from build123d import *

# Parameters (mm, degrees)
SKETCH1_R           = 2.38125
SKETCH1_R_2         = 14.2875
BOSS_EXTRUDE1_DEPTH = 6.35
FILLET1_R           = 12.7
SKETCH2_R           = 2.38125
CUT_EXTRUDE1_DEPTH  = 7.35
FILLET2_R           = 2.54


with BuildPart() as part:
    # Sketch1 → Boss-Extrude1 (new body)
    with BuildSketch(Plane(origin=(0, 0, 0), x_dir=(1, 0, 0), z_dir=(0, 1, 0))):
        Polygon((0, 0), (50.8, 0), (50.8, 127), (-25.4, 127), (-25.4, 50.8), (0, 50.8), align=None)
        with Locations((12.7, 12.7)):
            Circle(SKETCH1_R, mode=Mode.SUBTRACT)
        with Locations((25.4, 12.7)):
            Circle(SKETCH1_R, mode=Mode.SUBTRACT)
        with Locations((38.1, 12.7)):
            Circle(SKETCH1_R, mode=Mode.SUBTRACT)
        with Locations((25.4, 25.4)):
            Circle(SKETCH1_R, mode=Mode.SUBTRACT)
        with Locations((38.1, 25.4)):
            Circle(SKETCH1_R, mode=Mode.SUBTRACT)
        with Locations((25.4, 38.1)):
            Circle(SKETCH1_R, mode=Mode.SUBTRACT)
        with Locations((38.1, 38.1)):
            Circle(SKETCH1_R, mode=Mode.SUBTRACT)
        with Locations((12.7, 25.4)):
            Circle(SKETCH1_R, mode=Mode.SUBTRACT)
        with Locations((12.7, 38.1)):
            Circle(SKETCH1_R, mode=Mode.SUBTRACT)
        with Locations((6.35, 88.9)):
            Circle(SKETCH1_R_2, mode=Mode.SUBTRACT)
        with Locations((12.7, 50.8)):
            Circle(SKETCH1_R, mode=Mode.SUBTRACT)
        with Locations((25.4, 50.8)):
            Circle(SKETCH1_R, mode=Mode.SUBTRACT)
        with Locations((38.1, 50.8)):
            Circle(SKETCH1_R, mode=Mode.SUBTRACT)
    extrude(amount=BOSS_EXTRUDE1_DEPTH)

    # Fillet1
    fillet1_edges = [part.edges().sort_by_distance(p)[0] for p in [
        (-25.4, 3.175, -127),
        (50.8, 3.175, -127),
    ]]
    fillet(fillet1_edges, radius=FILLET1_R)

    # Sketch2 → Cut-Extrude1 (cut, through all)
    with BuildSketch(Plane(origin=(0, 6.35, 0), x_dir=(1, 0, 0), z_dir=(0, 1, 0))):
        with Locations((-19.05, 88.9)):
            Circle(SKETCH2_R)
        with Locations((-11.610512242, 106.860512242)):
            Circle(SKETCH2_R)
        with Locations((6.35, 114.3)):
            Circle(SKETCH2_R)
        with Locations((24.310512242, 106.860512242)):
            Circle(SKETCH2_R)
        with Locations((31.75, 88.9)):
            Circle(SKETCH2_R)
        with Locations((24.310512242, 70.939487758)):
            Circle(SKETCH2_R)
        with Locations((6.35, 63.5)):
            Circle(SKETCH2_R)
        with Locations((-11.610512242, 70.939487758)):
            Circle(SKETCH2_R)
    extrude(amount=-CUT_EXTRUDE1_DEPTH, mode=Mode.SUBTRACT)

    # Fillet2
    fillet2_edges = [part.edges().sort_by_distance(p)[0] for p in [
        (-25.4, 3.175, -50.8),
    ]]
    fillet(fillet2_edges, radius=FILLET2_R)


solid = part.part
Geometry check sheet. Reference: the model listing, model coordinates, mm. A direction names the side the tool comes from. Round coordinates to 2 decimals unless told otherwise and drop trailing zeros. Loops run counter-clockwise (first coordinate to the right, second up) from the corner with the lowest first, then second, coordinate; pieces in that order, holes last. Notation, with made-up numbers: (85.5, 38) - (93.5, 38) arc R28 cw to (93.5, 70) - close; hole circle Ø8 at (38, 59.25). An arc over 180 degrees is marked (long way). Answer as CSV lines item,"result".
(1) Depth check by flat-ended pin: pin 1 Ø4.5 at (x, z) = (12.7, -25.4) entering from +Y. Enter the tip coordinate at first touch or a pass-through.
Output values:
pin 1,"passes through"
(2) Cross-section at B-B, the plane z = -63.5. Enter the section's corners in (x, y), and give its area (3 significant figures).
Output values:
outline,"(-25.4, 0) - (3.97, 0) - (3.97, 6.35) - (-25.4, 6.35) - close; (8.73, 0) - (50.8, 0) - (50.8, 6.35) - (8.73, 6.35) - close"
area,"454 mm²"
(3) Cross-section at A-A, the plane x = 31.75. Enter the section's corners in (y, z).
Output values:
outline,"(0, -127) - (6.35, -127) - (6.35, -91.28) - (0, -91.28) - close; (0, -86.52) - (6.35, -86.52) - (6.35, 0) - (0, 0) - close"
(4) Cross-section at C-C, the plane z = -12.7. Enter the section's corners in (x, y).
Output values:
outline,"(0, 0) - (10.32, 0) - (10.32, 6.35) - (0, 6.35) - close; (15.08, 0) - (23.02, 0) - (23.02, 6.35) - (15.08, 6.35) - close; (27.78, 0) - (35.72, 0) - (35.72, 6.35) - (27.78, 6.35) - close; (40.48, 0) - (50.8, 0) - (50.8, 6.35) - (40.48, 6.35) - close"
(5) Release check for a two-part mould opening along X. For faces 1 (the face through (-24.636, 3.219, -51.524)), 2 (the face through (21, 6.35, -64)), 3 (the face through (12.39, 3.13, -53.16)) record: released by +X, released by -X, zero draft, split by the parting line, or undercut.
Output values:
face 1,"released by -X"
face 2,"zero draft"
face 3,"undercut"
(6) Set-up check for faces 4 (the face through (0, 3, -26)), 5 (the face through (14.97, 3.13, -26.12)): record each of +Z, -Z, +X, -X, +Y, -Y from which the full face is reachable in a straight line by a thin tool's end or side.
Output values:
face 4,"+Z, -X, +Y, -Y"
face 5,"+Y, -Y"
(7) Cross-section at D-D, the plane y = 2.5. Give the number of separate pieces and of enclosed holes in the cut face, and give its area (3 significant figures).
Output values:
separate pieces,"1"
enclosed holes,"21"
area,"7,320 mm²"
(8) Material ranges on line 1 along X through (y, z) = (2.5, -38.1); line 2 along Z through (x, y) = (38.1, 4.5); line 3 along Z through (x, y) = (6.35, 1.75), recorded low to high.
Output values:
line 1,"x = 0 to 10.32, 15.08 to 23.02, 27.78 to 35.72, 40.48 to 50.8"
line 2,"z = -127 to -53.18, -48.42 to -40.48, -35.72 to -27.78, -23.02 to -15.08, -10.32 to 0"
line 3,"z = -127 to -116.68, -111.92 to -103.19, -74.61 to -65.88, -61.12 to 0"
